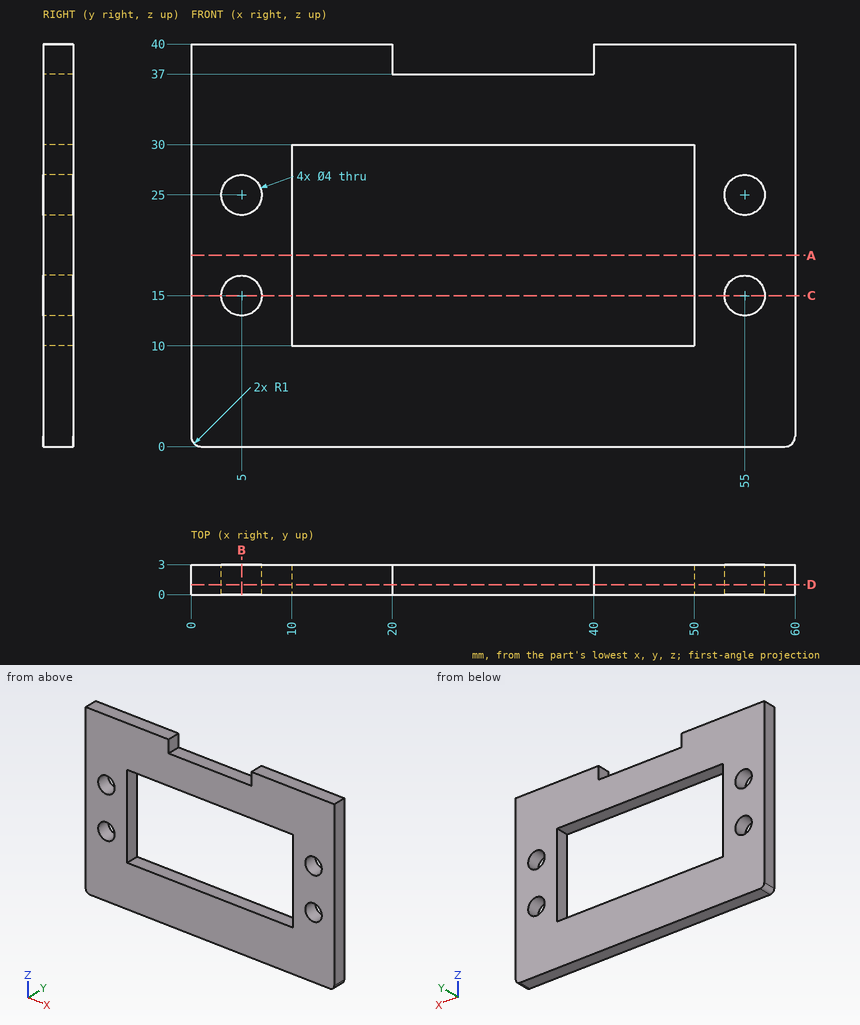
Verification items for this drawing (mm, ordinates from the low corner). Round coordinates to 2 decimals unless told otherwise and drop trailing zeros. Write each loop counter-clockwise with the first axis right and the second up, starting at its lowest first coordinate (ties: lowest second). Pieces come first, ordered by that corner, then holes. Notation, with made-up numbers: (-24, 67.25) - (11, 67.25) arc R8 ccw to (11, 75.25) - close; hole circle Ø7 at (-28.75, 69). An arc over 180 degrees is marked (long way). Answer as a JSON object with one key per item and string values. Group by question number.
Q1. Go/stop test with a flat-tipped pin: pin 1 Ø2.5 at (x, z) = (5, 25) entering from +Y. Record where the tip stops, or that it passes through.
Q2. Section check A-A, the plane z = 19. Enter the section's corners in (x, y), plus the area to 3 significant figures.
Q3. Section check C-C, the plane z = 15. Enter the section's corners in (x, y), plus the area to 3 significant figures.
Q4. Section check B-B, the plane x = 5. Enter the section's corners in (y, z).
Q5. Thickness scan on line 1 (X direction, y = 2.2, z = 25); line 2 (Z direction, x = 29, y = 2.4); line 3 (X direction, y = 2.35, z = 22.5). Record the ranges inside material, lowest first.
Q6. Section check D-D, the plane y = 1. Enter the section's corners in (x, z), plus the area to 3 significant figures.
Found:
{
 "1": {"pin 1": "passes through"},
 "2": {"outline": "(0, 0) - (10, 0) - (10, 3) - (0, 3) - close; (50, 0) - (60, 0) - (60, 3) - (50, 3) - close", "area": "60.0 mm^2"},
 "3": {"outline": "(0, 0) - (3, 0) - (3, 3) - (0, 3) - close; (7, 0) - (10, 0) - (10, 3) - (7, 3) - close; (50, 0) - (53, 0) - (53, 3) - (50, 3) - close; (57, 0) - (60, 0) - (60, 3) - (57, 3) - close", "area": "36.0 mm^2"},
 "4": {"outline": "(0, 0) - (3, 0) - (3, 13) - (0, 13) - close; (0, 17) - (3, 17) - (3, 23) - (0, 23) - close; (0, 27) - (3, 27) - (3, 40) - (0, 40) - close"},
 "5": {"line 1": "x = 0 to 3, 7 to 10, 50 to 53, 57 to 60", "line 2": "z = 0 to 10, 30 to 37", "line 3": "x = 0 to 10, 50 to 60"},
 "6": {"outline": "(0, 1) arc R1 ccw to (1, 0) - (59, 0) arc R1 ccw to (60, 1) - (60, 40) - (40, 40) - (40, 37) - (20, 37) - (20, 40) - (0, 40) - close; hole circle Ø4 at (5, 15); hole circle Ø4 at (5, 25); hole (10, 10) - (50, 10) - (50, 30) - (10, 30) - close; hole circle Ø4 at (55, 15); hole circle Ø4 at (55, 25)", "area": "1,490 mm^2"}
}
